from build123d import *

# Parameters (mm, degrees)
SKETCH1_R      = 1.49479
EXTRUDE1_DEPTH = 43.18
SKETCH2_R      = 0.9525
EXTRUDE2_DEPTH = 0.635
EXTRUDE3_START = 1.27
SKETCH3_R      = 1.49479
EXTRUDE3_DEPTH = 1.27
CHAMFER1_SIZE  = 0.508


with BuildPart() as part:
    # Sketch1 → Extrude1 (new body)
    with BuildSketch(Plane.XY):
        Circle(SKETCH1_R)
    extrude(amount=EXTRUDE1_DEPTH)

    # Sketch2 → Extrude2 (add)
    with BuildSketch(Plane(origin=(0, 0, 0), x_dir=(-1, 0, 0), z_dir=(0, 0, -1))):
        with Locations(Location((0, 0, 0), (0, 0, 180))):
            Circle(SKETCH2_R)
    extrude(amount=EXTRUDE2_DEPTH)

    # Sketch3 → Extrude3 (add)
    with BuildSketch(Plane(origin=(0, 0, -0.635), x_dir=(-1, 0, 0), z_dir=(0, 0, -1)).offset(EXTRUDE3_START)):
        with Locations(Location((0, 0, 0), (0, 0, 180))):
            Circle(SKETCH3_R)
    extrude(amount=-EXTRUDE3_DEPTH)

    # Chamfer1
    chamfer1_edges = [part.edges().sort_by_distance(p)[0] for p in [
        (-1.49479, 0, -1.905),
        (-1.49479, 0, 43.18),
    ]]
    chamfer(chamfer1_edges, length=CHAMFER1_SIZE)


solid = part.part
For this review, take the finished solid that the model builds, in its own axes (mm). Give positions to 0.01 mm unless a question says otherwise; leave off trailing zeros. Order: outer loops, then holes, each group sorted by start corner. A loop starts at its lowest first (then second) coordinate and runs counter-clockwise, first axis right, second up. Notation, with made-up numbers: M 45.5,72 L 103.5,72 A25 cw 103.5,104 Z; hole C 22.5,-13.5 d11. An arc over 180 degrees is marked long. Answer in a Markdown table with one row per item. Add a question column.
(1) Consider section A-A on z = 40. State the section outline as (x, y) points, and give its area (3 significant figures).
(2) Wall thickness on probe 1 along Z at (x, y) = (0.95, 0.25) (3 decimals); probe 2 along X at (y, z) = (-1.15, 4); probe 3 along Z at (x, y) = (0.85, 1) (3 decimals): over which ranges is each line inside the solid? List them lowest first. Write a range as [from, to].
(3) Mouldability with a two-part tool opening along Z and no side actions: class faces 1 (the face through (0, 0, 43.18)), 2 (the face through (-0.124, -0.944, -0.313)), 3 (the face through (0, 0, -1.905)) as +Z half, -Z half, draft (parallel to the pull), parting line (faces both ways), or undercut.
Evaluation:
| question | item | result |
|---|---|---|
| 1 | outline | C 0,0 d2.99 |
| 1 | area | 7.02 mm^2 |
| 2 | probe 1 | z = [-1.905, -0.635], [0, 43.18] |
| 2 | probe 2 | x = [-0.95, 0.95] |
| 2 | probe 3 | z = [-1.579, -0.635], [0, 42.854] |
| 3 | face 1 | +Z half |
| 3 | face 2 | undercut |
| 3 | face 3 | -Z half |
